```python
from build123d import *

# Parameters (mm, degrees)
SKETCH1_W                                           = 127
SKETCH1_H                                           = 50.8
BOSS_EXTRUDE1_DEPTH                                 = 50.8
F_7_16_0_4375_DIAMETER_HOLE2_D                      = 11.1125
F_7_16_0_4375_DIAMETER_HOLE2_DEPTH                  = 19.05
F_7_16_0_4375_DIAMETER_HOLE2_TIP                    = 3.338531814
CBORE_FOR_3_8_HEX_HEAD_BOLT1_D                      = 10.0838
CBORE_FOR_3_8_HEX_HEAD_BOLT1_CBORE_D                = 22.225
CBORE_FOR_3_8_HEX_HEAD_BOLT1_CBORE_DEPTH            = 6.8072
CSK_FOR_3_8_FLAT_HEAD_MACHINE_SCREW_100_D           = 10.0838
CSK_FOR_3_8_FLAT_HEAD_MACHINE_SCREW_100_DEPTH       = 38.1
CSK_FOR_3_8_FLAT_HEAD_MACHINE_SCREW_100_CSINK_D     = 19.3548
CSK_FOR_3_8_FLAT_HEAD_MACHINE_SCREW_100_CSINK_ANGLE = 100
CSK_FOR_3_8_FLAT_HEAD_MACHINE_SCREW_100_TIP         = 3.029479155
F_1_4_20_TAPPED_HOLE1_D                             = 5.1054
F_1_4_20_TAPPED_HOLE1_DEPTH                         = 25.4
F_1_4_20_TAPPED_HOLE1_CSINK_D                       = 7.62
F_1_4_20_TAPPED_HOLE1_CSINK_ANGLE                   = 100
F_1_4_20_TAPPED_HOLE1_TIP                           = 1.533816902


with BuildPart() as part:
    # Sketch1 → Boss-Extrude1 (new body)
    with BuildSketch(Plane.XY):
        Rectangle(SKETCH1_W, SKETCH1_H)
    extrude(amount=BOSS_EXTRUDE1_DEPTH)

    # 7/16 (0.4375) Diameter Hole2
    with Locations(Plane(origin=(-38.1, 25.4, 25.4), x_dir=(0, 0, 1), z_dir=(0, 1, 0))):
        with Locations((0, 0)):
            Hole(F_7_16_0_4375_DIAMETER_HOLE2_D / 2, depth=F_7_16_0_4375_DIAMETER_HOLE2_DEPTH)
            with Locations((0, 0, -(F_7_16_0_4375_DIAMETER_HOLE2_DEPTH + F_7_16_0_4375_DIAMETER_HOLE2_TIP / 2))):  # 118° drill point
                Cone(0, F_7_16_0_4375_DIAMETER_HOLE2_D / 2, F_7_16_0_4375_DIAMETER_HOLE2_TIP, mode=Mode.SUBTRACT)

    # CBORE for 3/8 Hex Head Bolt1 (through all)
    with Locations(Plane(origin=(-12.7, 25.4, 25.4), x_dir=(0, 0, 1), z_dir=(0, 1, 0))):
        with Locations((0, 0)):
            CounterBoreHole(CBORE_FOR_3_8_HEX_HEAD_BOLT1_D / 2, CBORE_FOR_3_8_HEX_HEAD_BOLT1_CBORE_D / 2, CBORE_FOR_3_8_HEX_HEAD_BOLT1_CBORE_DEPTH)

    # CSK for 3/8 Flat Head Machine Screw (100)1
    with Locations(Plane(origin=(12.7, 25.4, 25.4), x_dir=(0, 0, 1), z_dir=(0, 1, 0))):
        with Locations((0, 0)):
            CounterSinkHole(CSK_FOR_3_8_FLAT_HEAD_MACHINE_SCREW_100_D / 2, CSK_FOR_3_8_FLAT_HEAD_MACHINE_SCREW_100_CSINK_D / 2, depth=CSK_FOR_3_8_FLAT_HEAD_MACHINE_SCREW_100_DEPTH, counter_sink_angle=CSK_FOR_3_8_FLAT_HEAD_MACHINE_SCREW_100_CSINK_ANGLE)
            with Locations((0, 0, -(CSK_FOR_3_8_FLAT_HEAD_MACHINE_SCREW_100_DEPTH + CSK_FOR_3_8_FLAT_HEAD_MACHINE_SCREW_100_TIP / 2))):  # 118° drill point
                Cone(0, CSK_FOR_3_8_FLAT_HEAD_MACHINE_SCREW_100_D / 2, CSK_FOR_3_8_FLAT_HEAD_MACHINE_SCREW_100_TIP, mode=Mode.SUBTRACT)

    # 1/4-20 Tapped Hole1
    with Locations(Plane(origin=(38.1, 25.4, 25.4), x_dir=(0, 0, 1), z_dir=(0, 1, 0))):
        with Locations((0, 0)):
            CounterSinkHole(F_1_4_20_TAPPED_HOLE1_D / 2, F_1_4_20_TAPPED_HOLE1_CSINK_D / 2, depth=F_1_4_20_TAPPED_HOLE1_DEPTH, counter_sink_angle=F_1_4_20_TAPPED_HOLE1_CSINK_ANGLE)
            with Locations((0, 0, -(F_1_4_20_TAPPED_HOLE1_DEPTH + F_1_4_20_TAPPED_HOLE1_TIP / 2))):  # 118° drill point
                Cone(0, F_1_4_20_TAPPED_HOLE1_D / 2, F_1_4_20_TAPPED_HOLE1_TIP, mode=Mode.SUBTRACT)


solid = part.part
```
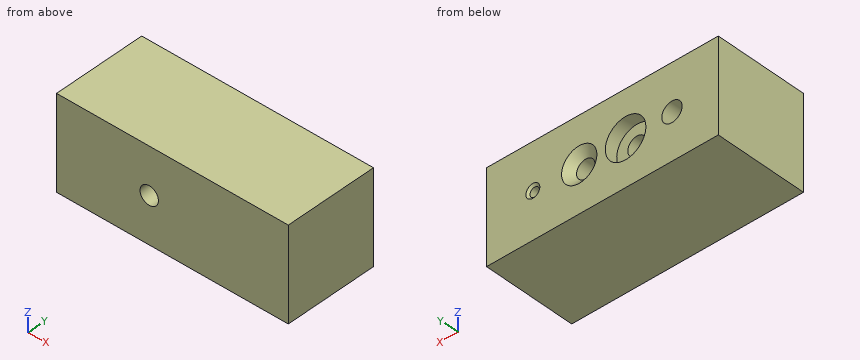
Here's how the part is built. I have some questions about the finished solid (model axes, mm). Give positions to 0.01 mm unless a question says otherwise; leave off trailing zeros. Loops run counter-clockwise (first coordinate to the right, second up) from the corner with the lowest first, then second, coordinate; pieces in that order, holes last. Notation, with made-up numbers: M -9,0 L 35,0 A24 ccw 35,14 Z; hole C 60.5,-35 d11. An arc over 180 degrees is marked long. Use one line per item in the form item = value. Start each with the question number.
Q1. If we section it at A-A (y = 16): Write out the boundary of the cut face in (x, z).
Q2. If we section it at B-B (x = -12.7): Write out the boundary of the cut face in (y, z), then the cut area to 3 significant figures.
Q3. If we section it at C-C (y = -10): Write out the boundary of the cut face in (x, z), then the cut area to 3 significant figures.
Q4. Will these pins go through, and if not, where does the flat tip stop? pin 1 Ø8 at (x, z) = (12.7, 25.4) entering from +Y; pin 2 Ø4 at (x, z) = (38.1, 25.4) entering from +Y.
Q5. I need wall thicknesses on line 1 along X through (y, z) = (-5, 25); line 2 along X through (y, z) = (12, 25.4); line 3 along Z through (x, y) = (-38.1, 18). Which ranges of each line are inside material? Lowest first, please.
Taken from the geometry:
q1.outline = M -63.5,0 L 63.5,0 L 63.5,50.8 L -63.5,50.8 Z; hole C -38.1,25.4 d11.11; hole C -12.7,25.4 d10.08; hole C 12.7,25.4 d10.08; hole C 38.1,25.4 d5.11
q2.outline = M -25.4,0 L 25.4,0 L 25.4,14.29 L 18.59,14.29 L 18.59,20.36 L -25.4,20.36 Z; M -25.4,30.44 L 18.59,30.44 L 18.59,36.51 L 25.4,36.51 L 25.4,50.8 L -25.4,50.8 Z
q2.area = 1,990 mm^2
q3.outline = M -63.5,0 L 63.5,0 L 63.5,50.8 L -63.5,50.8 Z; hole C -12.7,25.4 d10.08; hole C 12.7,25.4 d10.08
q3.area = 6,290 mm^2
q4.pin_1 = -13.33
q4.pin_2 = -0.33
q5.line_1 = -63.5 to -17.73, -7.67 to 7.67, 17.73 to 63.5
q5.line_2 = -63.5 to -43.66, -32.54 to -17.74, -7.66 to 7.66, 17.74 to 35.55, 40.65 to 63.5
q5.line_3 = 0 to 19.84, 30.96 to 50.8
